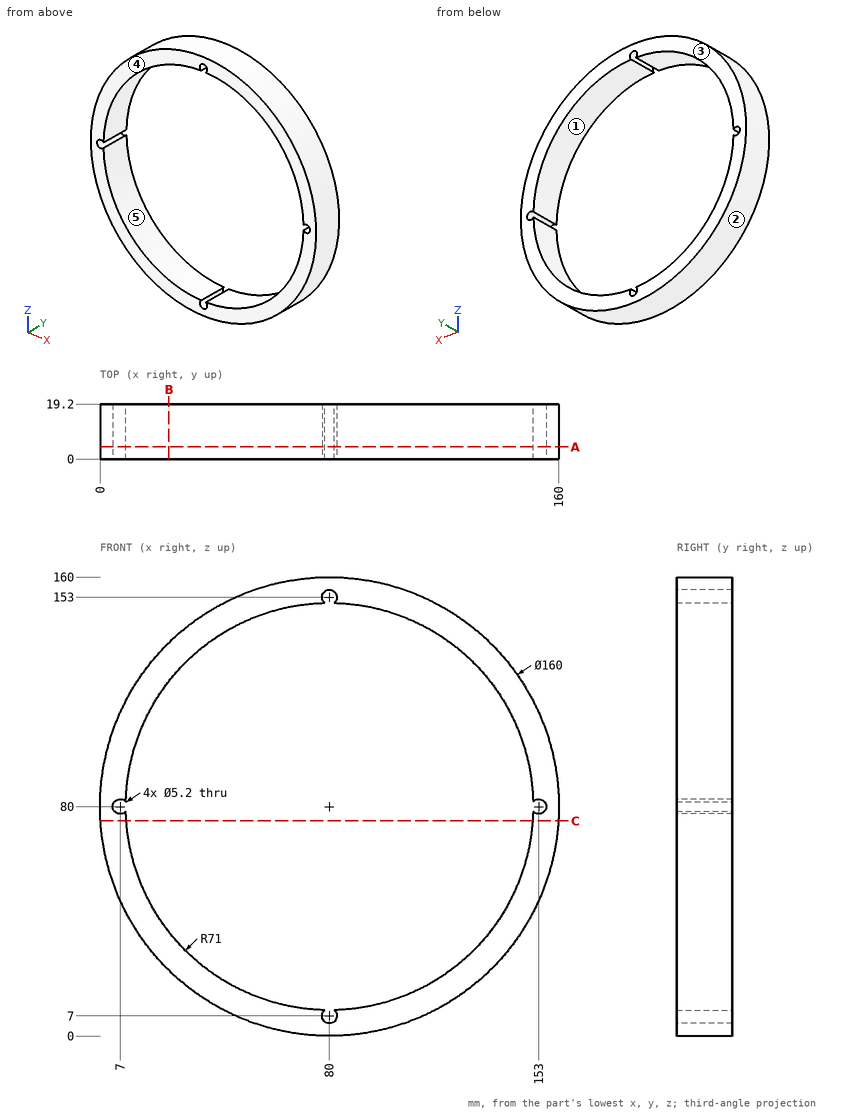
Source: three-view drawing plus pictorial views. Frame: mm from the lowest corner of the part. A direction names the side the tool comes from. Round coordinates to 2 decimals unless told otherwise and drop trailing zeros. Write each loop counter-clockwise with the first axis right and the second up, starting at its lowest first coordinate (ties: lowest second). Pieces come first, ordered by that corner, then holes. Notation, with made-up numbers: (3.5, 11) -> (12.5, 11) arc R20 ccw to (12.5, 20) -> close; hole circle Ø3 at (64.5, 8.5). An arc over 180 degrees is marked (long way). Return JSON: item names as keys, results as strings.
Q1. Mould query, pull axis Z, two halves, no side actions, for the marked faces 1, 2 and 3. Classes: +Z half, -Z half, draft (parallel to the pull), parting line (faces both ways), or undercut.
From the geometry:
{"face 1": "undercut", "face 2": "parting line", "face 3": "draft"}
Q2. Section B-B on x = 24. Return the cut outline in (y, z).
From the geometry:
{"outline": "(0, 22.87) -> (19.2, 22.87) -> (19.2, 36.35) -> (0, 36.35) -> close; (0, 123.65) -> (19.2, 123.65) -> (19.2, 137.13) -> (0, 137.13) -> close"}
Q3. Section A-A on y = 4.25. Return the cut outline in (x, z).
From the geometry:
{"outline": "circle Ø160 at (80, 80); hole (9.02, 78.36) arc R71 ccw to (78.36, 9.02) arc R2.6 ccw (long way) to (81.64, 9.02) arc R71 ccw to (150.98, 78.36) arc R2.6 ccw (long way) to (150.98, 81.64) arc R71 ccw to (81.64, 150.98) arc R2.6 ccw (long way) to (78.36, 150.98) arc R71 ccw to (9.02, 81.64) arc R2.6 ccw (long way) to start"}
Q4. First-contact query: pin 1 Ø4 at (x, y) = (60.5, 7) entering from +Z; pin 2 Ø5 at (y, z) = (11.5, 67.5) entering from +X; pin 3 Ø5 at (x, y) = (43, 15) entering from -Z. Flat tips, straight axial feed; report the tip coordinate or a pass-through.
From the geometry:
{"pin 1": "z = 158.06", "pin 2": "x = 159.37", "pin 3": "z = 7.82"}
Q5. Set-up query: the marked faces 4 and 5. Return all of +Z, -Z, +X, -X, +Y, -Y with unobstructed straight access to the full face (end or side cutting, diameter ignored); none if empty.
From the geometry:
{"face 4": "+Z, -Z, +X, -X, -Y", "face 5": "+Y, -Y"}
Q6. Section C-C on z = 75. Return the cut outline in (x, y).
From the geometry:
{"outline": "(0.16, 0) -> (9.18, 0) -> (9.18, 19.2) -> (0.16, 19.2) -> close; (150.82, 0) -> (159.84, 0) -> (159.84, 19.2) -> (150.82, 19.2) -> close"}
Q7. Ray query, line 1 (Z direction, x = 45.5, y = 16); line 2 (Z direction, x = 58, y = 3.25); line 3 (X direction, y = 6.5, z = 153). Return the intervals inside material, ascending.
From the geometry:
{"line 1": "7.82 to 17.95, 142.05 to 152.18", "line 2": "3.08 to 12.49, 147.51 to 156.92", "line 3": "47.27 to 77.4, 82.6 to 112.73"}
